from build123d import *

# Parameters (mm, degrees)
F1_DEPTH      = 4
F1_DEPTH_BACK = 4
F2_COUNT      = 14


with BuildPart() as f1:
    # F0 (on Front) → F1 (new body, two sides)
    with BuildSketch(Plane.XZ) as f1_sk:
        Polygon((0, 0.5), (0, 0), (8.40777345, 0), (17.7297703922, 24.8893443495), (17.1958512824, 24.8893443495), (8.0611231732, 0.5), align=None)
    extrude(amount=F1_DEPTH)
    extrude(f1_sk.sketch, amount=-F1_DEPTH_BACK)

    # F2: F1 ×14 about axis
    f2_axis = Axis((0, 0, 1.0500000276), (0, 0, -1))


with BuildPart() as f1_1:
    add(f1.part)
    for i in range(1, F2_COUNT):
        add(f1.part.rotate(f2_axis, i * 360 / F2_COUNT))


solid = f1_1.part
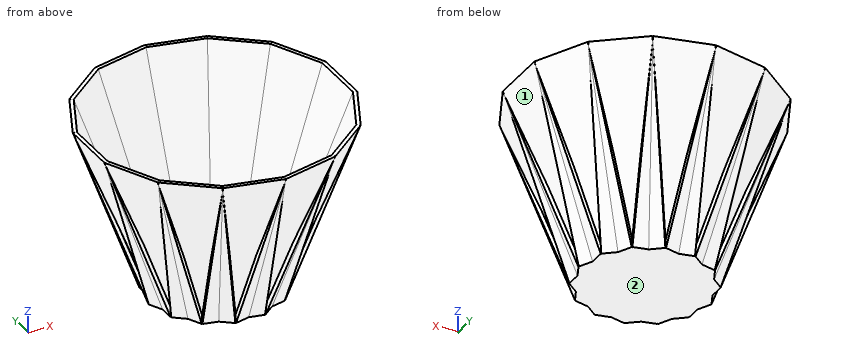
Could you check a few things on this model? Use its own coordinates, in mm. Face numbers are marked on the shaded views. Coordinates: 2 decimals unless noted, no trailing zeros. One line per question, with ' | ' between items.
1) If we mould it in two halves opening along Y, with no side actions, what happens to the marked faces 1 and 2? For each: released by +Y, released by -Y, zero draft, split by the parting line, or undercut.
Checks:
face 1: undercut | face 2: zero draft
2) For pin 1 Ø10 at (y, z) = (-13.5, 14) entering from +X; pin 2 Ø2 at (x, z) = (-4, 21.5) entering from +Y; pin 3 Ø6 at (x, z) = (-14, 21.5) entering from +Y; pin 4 Ø10 at (x, y) = (6.5, -0.5) entering from -Z, each with a flat end and sliding along its axis, tell me the tip position at first contact or that it passes through.
Checks:
pin 1: x = 11.92 | pin 2: y = 16.42 | pin 3: y = 12.68 | pin 4: z = 0
3) I need wall thicknesses on probe 1 along Z at (x, y) = (-5, 5); probe 2 along Y at (x, z) = (-8, 23.5); probe 3 along X at (y, z) = (-14.5, 21.5). Which ranges of each line are inside material? Lowest first, please. Write a range as [from, to].
Checks:
probe 1: [0, 0.5] | probe 2: [-15.63, -14.95], [14.95, 15.63] | probe 3: [-8.22, -7.36], [7.36, 8.22]
